Work out the finished part from the listing and answer in its coordinate system (mm). Round coordinates to 2 decimals unless told otherwise and drop trailing zeros. Loops run counter-clockwise (first coordinate to the right, second up) from the corner with the lowest first, then second, coordinate; pieces in that order, holes last.
Autodesk Inventor part; units mm, degrees
ref_plane "YZ Plane" through (0, 0, 0) normal (1, 0, 0) x (0, 1, 0)
ref_plane "XZ Plane" through (0, 0, 0) normal (0, 1, 0) x (-1, 0, 0)
ref_plane "XY Plane" through (0, 0, 0) normal (0, 0, 1) x (1, 0, 0)
sketch "Sketch1" plane through (0, 0, 0) normal (0, 1, 0) x (-1, 0, 0)
  line L0 (-85, 43) -> (-85, -43)
  line L1 (85, -43) -> (85, 43)
  arc A0 (-115.5144, -47.7642) -> (115.5144, -47.7642) centre (0, 0) ccw
  arc A1 (115.5144, 47.7642) -> (-115.5144, 47.7642) centre (0, 0) ccw
  line L2 (113.6662, 45) -> (87, 45)
  line L3 (-87, 45) -> (-113.6662, 45)
  line L4 (87, -45) -> (113.6662, -45)
  line L5 (-113.6662, -45) -> (-87, -45)
  circle A2 centre (63, -8) radius 1.5
  circle A3 centre (63, 8) radius 1.5
  circle A4 centre (77, 8) radius 1.5
  circle A5 centre (77, -8) radius 1.5
  circle A6 centre (-63, -8) radius 1.5
  circle A7 centre (-63, 8) radius 1.5
  circle A8 centre (-77, 8) radius 1.5
  circle A9 centre (-77, -8) radius 1.5
  circle A10 centre (70, -90) radius 1.5
  circle A11 centre (-70, -90) radius 1.5
  circle A12 centre (-70, 90) radius 1.5
  circle A13 centre (70, 90) radius 1.5
  line L6 (13, 15) -> (-13, 15)
  line L7 (-15, 13) -> (-15, -13)
  line L8 (-13, -15) -> (13, -15)
  line L9 (15, -13) -> (15, 13)
  circle A14 centre (-18.5, -51.5) radius 1.5
  circle A15 centre (-18.5, -88.5) radius 1.5
  circle A16 centre (18.5, -88.5) radius 1.5
  circle A17 centre (18.5, -51.5) radius 1.5
  arc A18 (115.5144, -47.7642) -> (113.6662, -45) centre (113.6662, -47) ccw
  arc A19 (85, -43) -> (87, -45) centre (87, -43) ccw
  arc A20 (87, 45) -> (85, 43) centre (87, 43) ccw
  arc A21 (113.6662, 45) -> (115.5144, 47.7642) centre (113.6662, 47) ccw
  arc A22 (-115.5144, 47.7642) -> (-113.6662, 45) centre (-113.6662, 47) ccw
  arc A23 (-85, 43) -> (-87, 45) centre (-87, 43) ccw
  arc A24 (-87, -45) -> (-85, -43) centre (-87, -43) ccw
  arc A25 (-113.6662, -45) -> (-115.5144, -47.7642) centre (-113.6662, -47) ccw
  arc A26 (-15, -13) -> (-13, -15) centre (-13, -13) ccw
  arc A27 (-13, 15) -> (-15, 13) centre (-13, 13) ccw
  arc A28 (15, 13) -> (13, 15) centre (13, 13) ccw
  arc A29 (13, -15) -> (15, -13) centre (13, -13) ccw
  circle A30 centre (-19.5, -99.2842) radius 2
  circle A31 centre (19.5, -99.2842) radius 2
  circle A32 centre (-19.5, 99.2842) radius 2
  circle A33 centre (19.5, 99.2842) radius 2
  point P0 (116.619, -45)
  point P1 (116.619, 45)
  point P2 (-116.619, 45)
  point P3 (-116.619, -45)
  point P4 (85, 0)
extrude "Extrusion2" add sketch "Sketch1" along normal blind 3
1. Consider probe 1 along Z at (x, y) = (77, 0.6); probe 2 along Z at (x, y) = (63, 2.35); probe 3 along X at (y, z) = (0.75, 90). Determine where each line is inside the solid, lowest interval first.
Answer key:
probe 1: z = -98.47 to -9.5, -6.5 to 6.5, 9.5 to 98.47
probe 2: z = -107.96 to -9.5, -6.5 to 6.5, 9.5 to 107.96
probe 3: x = -86.75 to -71.5, -68.5 to 68.5, 71.5 to 86.75
2. Given pin 1 (1.8 mm diameter, centred on x = 18.5, z = -51.5, fed in from +Y); pin 2 (0.9 mm diameter, centred on x = -104.5, y = 1, fed in from +Z), each flat-ended and moving along its own axis, determine where each tip first touches the part or whether it passes through.
Answer key:
pin 1: passes through
pin 2: stops at z = 69.27
3. Find section D-D (y = 1.1). Give the number of separate pieces and of enclosed holes in the cut face, then the cut area to 3 significant figures.
Answer key:
separate pieces: 1
enclosed holes: 21
area: 41,300 mm2
4. Find section B-B (z = 57). Write down the section's boundary in (x, y).
Answer key:
outline: (-111.25, 0) - (111.25, 0) - (111.25, 3) - (-111.25, 3) - close
5. Find section A-A (x = 101.5). Write down the section's boundary in (y, z).
Answer key:
outline: (0, -72.96) - (3, -72.96) - (3, -45) - (0, -45) - close; (0, 45) - (3, 45) - (3, 72.96) - (0, 72.96) - close
6. Find section C-C (x = -56.5). Write down the section's boundary in (y, z), then the cut area to 3 significant figures.
Answer key:
outline: (0, -111.5) - (3, -111.5) - (3, 111.5) - (0, 111.5) - close
area: 669 mm2
